Build history of the part. All positions in model axes, mm. A direction names the side the tool comes from. Give positions to 0.01 mm unless a question says otherwise; leave off trailing zeros. Order: outer loops, then holes, each group sorted by start corner. A loop starts at its lowest first (then second) coordinate and runs counter-clockwise, first axis right, second up. Notation, with made-up numbers: (-1, 24) - (8, 24) arc R7 cw to (8, 30) - close; hole circle Ø7 at (11, 36). An arc over 180 degrees is marked (long way). Use a Markdown table: item, result.
from build123d import *

# Parameters (mm, degrees)
F1_DEPTH = 6


with BuildPart() as f1:
    # F0 (on Top) → F1 (new body)
    with BuildSketch(Plane.XY):
        with BuildLine():
            Line((5.233688, 8), (0, 8))
            Line((0, 8), (-17.233688, 8))
            ThreePointArc((-17.233688, 8), (-19, 0), (-17.233688, -8))
            Line((-17.233688, -8), (5.233688, -8))
            ThreePointArc((5.233688, -8), (7, 0), (5.233688, 8))
        make_face()
        Polygon((-9, 3), (-9, 0), (-9, -3), (-15, -3), (-15, 3), align=None, mode=Mode.SUBTRACT)
        with BuildLine():
            ThreePointArc((0, 3), (2.12132, 2.12132), (3, 0))
            ThreePointArc((3, 0), (0, -3), (-3, 0))
            ThreePointArc((-3, 0), (-2.12132, 2.12132), (0, 3))
        make_face(mode=Mode.SUBTRACT)
    extrude(amount=F1_DEPTH)


solid = f1.part
1) Tool access for faces 1 (the flat face through (-6, 0, 0)), 2 (the flat face through (-15, 0, 3)): list every direction of +Z, -Z, +X, -X, +Y, -Y with a clear straight run to the whole face (end or side of a thin tool).
Computed:
| item | result |
|---|---|
| face 1 | -Z, +X, -X, +Y, -Y |
| face 2 | +Z, -Z |
2) Slice it at B-B (y = 0.75). Write the cut outline in (x, z).
Computed:
| item | result |
|---|---|
| outline | (-18.99, 0) - (-15, 0) - (-15, 6) - (-18.99, 6) - close; (-9, 0) - (-2.9, 0) - (-2.9, 6) - (-9, 6) - close; (2.9, 0) - (6.99, 0) - (6.99, 6) - (2.9, 6) - close |
3) Slice it at C-C (y = 4). Write the cut outline in (x, z).
Computed:
| item | result |
|---|---|
| outline | (-18.57, 0) - (6.57, 0) - (6.57, 6) - (-18.57, 6) - close |
4) Wall check: line 1 (X direction, y = 2.5, z = 1.65); line 2 (Y direction, x = -11.5, z = 0.7); line 3 (X direction, y = -0.75, z = 2.2). Give the ranges that are in metal, low to high. Write a range as from..to.
Computed:
| item | result |
|---|---|
| line 1 | x = -18.83..-15, -9..-1.66, 1.66..6.83 |
| line 2 | y = -8..-3, 3..8 |
| line 3 | x = -18.99..-15, -9..-2.9, 2.9..6.99 |
5) Slice it at D-D (y = -6). Write the cut outline in (x, z).
Computed:
| item | result |
|---|---|
| outline | (-18.03, 0) - (6.03, 0) - (6.03, 6) - (-18.03, 6) - close |
6) Slice it at A-A (z = 2.55). Write the cut outline in (x, y).
Computed:
| item | result |
|---|---|
| outline | (-17.23, -8) - (5.23, -8) arc R19 ccw to (5.23, 8) - (-17.23, 8) arc R19 ccw to start; hole (-15, -3) - (-9, -3) - (-9, 3) - (-15, 3) - close; hole (-3, 0) arc R3 ccw to (3, 0) arc R3 ccw to (0, 3) arc R3 ccw to start |
7) Pin check, flat tip, straight feed: P1, Ø2, axis at y = 1.5, z = 4, coming from the -X side. Stop position of the tip, or through.
Computed:
| item | result |
|---|---|
| P1 | stops at x = -18.99 |
8) Two-plate mould, pull along Y, no slides. Class faces 3 (the flat face through (-12, 3, 3)), 4 (the flat face through (-6, -8, 3)), 5 (the cylindrical face through (-19, 0, 3)), 6 (the flat face through (-9, 0, 3)): +Y half, -Y half, draft (parallel to the pull), parting line (faces both ways), or undercut.
Computed:
| item | result |
|---|---|
| face 3 | undercut |
| face 4 | -Y half |
| face 5 | parting line |
| face 6 | undercut |
